```python
from build123d import *

# Parameters (mm, degrees)
EXTRUDE_1_DEPTH     = 10
SKETCH_2_W          = 10
SKETCH_2_H          = 510
EXTRUDE_2_DEPTH     = 500
EXTRUDE_3_DEPTH     = 10
EXTRUDE_4_DEPTH     = 190
SKETCH_5_W          = 640
SKETCH_5_H          = 10
EXTRUDE_5_DEPTH     = 200
CUT_EXTRUDE_1_DEPTH = 20
SKETCH_7_W          = 523.996532841
SKETCH_7_H          = 100
EXTRUDE_7_DEPTH     = 10
EXTRUDE_8_DEPTH     = 100
EXTRUDE_9_DEPTH     = 10
EXTRUDE_10_DEPTH    = 10
SKETCH_11_W         = 810
SKETCH_11_H         = 510
EXTRUDE_11_DEPTH    = 10
SKETCH_12_W         = 520
SKETCH_12_H         = 510
CUT_EXTRUDE_2_DEPTH = 120
SKETCH_13_W         = 520
SKETCH_13_H         = 510
CUT_EXTRUDE_3_DEPTH = 50
EXTRUDE_12_DEPTH    = 10
SKETCH_15_W         = 520
SKETCH_15_H         = 510
EXTRUDE_13_DEPTH    = 10
EXTRUDE_15_DEPTH    = 100
SKETCH_18_W         = 660
SKETCH_18_H         = 520
SKETCH_18_W_2       = 640
SKETCH_18_H_2       = 500
EXTRUDE_16_DEPTH    = 120
SKETCH_19_W         = 400
SKETCH_19_H         = 12
EXTRUDE_17_DEPTH    = 480
SKETCH_20_W         = 330
SKETCH_20_H         = 15
EXTRUDE_18_DEPTH    = 230


with BuildPart() as part:
    # 草图1 → 凸台-拉伸1 (new body)
    with BuildSketch(Plane(origin=(0, 0, 0), x_dir=(1, 0, 0), z_dir=(0, 1, 0))):
        Polygon((0, 300), (0, 510), (160, 510), (160, 320), (800, 320), (800, 0), (0, 0), align=None)
    extrude(amount=EXTRUDE_1_DEPTH)

    # 草图2 → 凸台-拉伸2 (add)
    with BuildSketch(Plane(origin=(0, 10, 0), x_dir=(1, 0, 0), z_dir=(0, 1, 0))):
        with Locations((5, 255)):
            Rectangle(SKETCH_2_W, SKETCH_2_H)
    extrude(amount=EXTRUDE_2_DEPTH)

    # 草图3 → 凸台-拉伸3 (add)
    with BuildSketch(Plane(origin=(0, 0, -510), x_dir=(-1, 0, 0), z_dir=(0, 0, -1))):
        Polygon((-10, 510), (-10, 10), (-160, 10), (-450.008667897, 510), align=None)
    extrude(amount=-EXTRUDE_3_DEPTH)

    # 草图4 → 凸台-拉伸4 (add)
    with BuildSketch(Plane(origin=(0, 0, -510), x_dir=(-1, 0, 0), z_dir=(0, 0, -1))):
        Polygon((-276.003467159, 210), (-160, 10), (-160, 0), (-169.762228515, 0), (-169.762228515, 10), (-285.765695674, 210), align=None)
    extrude(amount=-EXTRUDE_4_DEPTH)

    # 草图5 → 凸台-拉伸5 (add)
    with BuildSketch(Plane(origin=(0, 10, 0), x_dir=(1, 0, 0), z_dir=(0, 1, 0))):
        with Locations((480, 315)):
            Rectangle(SKETCH_5_W, SKETCH_5_H)
    extrude(amount=EXTRUDE_5_DEPTH)

    # 草图6 → 切除-拉伸1 (cut)
    with BuildSketch(Plane(origin=(0, 0, -320), x_dir=(-1, 0, 0), z_dir=(0, 0, -1))):
        Polygon((-160, 210), (-276.003467159, 210), (-160, 10), align=None)
    extrude(amount=-CUT_EXTRUDE_1_DEPTH, mode=Mode.SUBTRACT)

    # 草图7 → 凸台-拉伸7 (add)
    with BuildSketch(Plane(origin=(0, 210, 0), x_dir=(1, 0, 0), z_dir=(0, 1, 0))):
        with Locations((538.00173358, 360)):
            Rectangle(SKETCH_7_W, SKETCH_7_H)
    extrude(amount=-EXTRUDE_7_DEPTH)

    # 草图8 → 凸台-拉伸8 (add)
    with BuildSketch(Plane(origin=(0, 0, -510), x_dir=(-1, 0, 0), z_dir=(0, 0, -1))):
        Polygon((-276.003467159, 210), (-450.008667897, 510), (-459.770896412, 510), (-285.765695674, 210), align=None)
    extrude(amount=-EXTRUDE_8_DEPTH)

    # 草图9 → 凸台-拉伸9 (add)
    with BuildSketch(Plane.XY.offset(-410)):
        Polygon((276.003467159, 210), (450.008667897, 510), (800, 510), (800, 210), align=None)
    extrude(amount=EXTRUDE_9_DEPTH)

    # 草图10 → 凸台-拉伸10 (add)
    with BuildSketch(Plane(origin=(800, 0, 0), x_dir=(0, 0, -1), z_dir=(1, 0, 0))):
        Polygon((0, 0), (320, 0), (320, 200), (410, 200), (410, 510), (0, 510), align=None)
    extrude(amount=EXTRUDE_10_DEPTH)

    # 草图11 → 凸台-拉伸11 (add)
    with BuildSketch(Plane.XY):
        with Locations((405, 255)):
            Rectangle(SKETCH_11_W, SKETCH_11_H)
    extrude(amount=EXTRUDE_11_DEPTH)

    # 草图12 → 切除-拉伸2 (cut)
    with BuildSketch(Plane.ZY):
        with Locations((-250, 255)):
            Rectangle(SKETCH_12_W, SKETCH_12_H)
    extrude(amount=-CUT_EXTRUDE_2_DEPTH, mode=Mode.SUBTRACT)

    # 草图13 → 切除-拉伸3 (cut)
    with BuildSketch(Plane(origin=(810, 0, 0), x_dir=(0, 0, -1), z_dir=(1, 0, 0))):
        with Locations((250, 255)):
            Rectangle(SKETCH_13_W, SKETCH_13_H)
    extrude(amount=-CUT_EXTRUDE_3_DEPTH, mode=Mode.SUBTRACT)

    # 草图14 → 凸台-拉伸12 (add)
    with BuildSketch(Plane(origin=(760, 0, 0), x_dir=(0, 0, -1), z_dir=(1, 0, 0))):
        Polygon((-10, 510), (320, 510), (410, 510), (410, 200), (320, 200), (320, 0), (-10, 0), align=None)
    extrude(amount=EXTRUDE_12_DEPTH)

    # 草图15 → 凸台-拉伸13 (add)
    with BuildSketch(Plane.ZY.offset(-120)):
        with Locations((-250, 255)):
            Rectangle(SKETCH_15_W, SKETCH_15_H)
    extrude(amount=EXTRUDE_13_DEPTH)

    # 草图17 → 凸台-拉伸15 (add)
    with BuildSketch(Plane(origin=(0, 0, -410), x_dir=(-1, 0, 0), z_dir=(0, 0, -1))):
        Polygon((-770, 510), (-459.770896412, 510), (-453.970723054, 500), (-770, 500), align=None)
    extrude(amount=EXTRUDE_15_DEPTH)

    # 草图18 → 凸台-拉伸16 (add)
    with BuildSketch(Plane(origin=(0, 510, 0), x_dir=(1, 0, 0), z_dir=(0, 1, 0))):
        with Locations((440, 250)):
            Rectangle(SKETCH_18_W, SKETCH_18_H)
        with Locations((440, 250)):
            Rectangle(SKETCH_18_W_2, SKETCH_18_H_2, mode=Mode.SUBTRACT)
    extrude(amount=EXTRUDE_16_DEPTH)

    # 草图19 → 凸台-拉伸17 (add)
    with BuildSketch(Plane.ZY.offset(-110)):
        with Locations((-250, 506)):
            Rectangle(SKETCH_19_W, SKETCH_19_H)
    extrude(amount=EXTRUDE_17_DEPTH)

    # 草图20 → 凸台-拉伸18 (add)
    with BuildSketch(Plane(origin=(770, 0, 0), x_dir=(0, 0, -1), z_dir=(1, 0, 0))):
        with Locations((155, 207.5)):
            Rectangle(SKETCH_20_W, SKETCH_20_H)
    extrude(amount=EXTRUDE_18_DEPTH)


solid = part.part
```
Verification items for the finished model (mm, model axes). A direction names the side the tool comes from. Give positions to 0.01 mm unless a question says otherwise; leave off trailing zeros. Write each loop counter-clockwise with the first axis right and the second up, starting at its lowest first coordinate (ties: lowest second). Pieces come first, ordered by that corner, then holes. Notation, with made-up numbers: M -32.75,49.5 L 20.25,49.5 A13 cw 20.25,58.5 Z; hole C 45.5,-30 d8. An arc over 180 degrees is marked long. One line per question, with ' | ' between items.
1) Set-up check for faces 1 (the flat face through (607, 510, -449)), 2 (the flat face through (-127, 500, -253)), 3 (the flat face through (-127, 512, -253)), 4 (the flat face through (576, 352, -410)), 5 (the flat face through (883, 215, -153)): record each of +Z, -Z, +X, -X, +Y, -Y from which the full face is reachable in a straight line by a thin tool's end or side.
Result:
face 1: +Y | face 2: +Z, -Z, -X, -Y | face 3: +Z, -Z, -X, +Y | face 4: -Z, +X, -Y | face 5: +Z, -Z, +X, +Y
2) Mould release check, pull along X, two halves, no side actions. Record for faces 6 (the flat face through (575, 362, -400)), 7 (the flat face through (466, 101, -320)): released by +X, released by -X, zero draft, split by the parting line, or undercut.
Result:
face 6: undercut | face 7: zero draft
3) Section check D-D on z = -138.5. Enter the section's corners in (x, y), plus the area to 3 significant figures.
Result:
outline: M -370,500 L 110,500 L 110,0 L 770,0 L 770,200 L 1000,200 L 1000,215 L 770,215 L 770,630 L 760,630 L 760,10 L 120,10 L 120,630 L 110,630 L 110,512 L -370,512 Z | area: 28,200 mm2
4) Gauge pin test, flat ends, axial feed: pin 1 Ø2 at (x, z) = (-185.5, -178) entering from -Y; pin 2 Ø5 at (y, z) = (475, -168.5) entering from -X; pin 3 Ø9.5 at (x, y) = (-167, 504.5) entering from +Z; pin 4 Ø2 at (x, z) = (226.5, -175) entering from -Y. Record the tip position at first contact, or that the pin passes through.
Result:
pin 1: stops at y = 500 | pin 2: stops at x = 110 | pin 3: stops at z = -50 | pin 4: stops at y = 0
5) Section check A-A on z = -364.5. Enter the section's corners in (x, y).
Result:
outline: M -370,500 L 110,500 L 110,0 L 169.76,0 L 169.76,10 L 279.97,200 L 770,200 L 770,630 L 760,630 L 760,210 L 276,210 L 160,10 L 120,10 L 120,630 L 110,630 L 110,512 L -370,512 Z
6) Thickness scan on line 1 along X through (y, z) = (305.5, -143); line 2 along Z through (x, y) = (415.5, 339); line 3 along Z through (x, y) = (129, 409). Record the ranges inside material, lowest first. Write a range as [from, to].
Result:
line 1: x = [110, 120], [760, 770] | line 2: z = [-410, -400], [0, 10] | line 3: z = [-510, -500], [0, 10]
7) Section check B-B on y = 434. Enter the section's corners in (x, z), plus the area to 3 significant figures.
Result:
outline: M 110,-510 L 415.69,-510 L 415.69,-410 L 770,-410 L 770,10 L 110,10 Z; hole M 120,-500 L 405.93,-500 L 405.93,-400 L 760,-400 L 760,0 L 120,0 Z | area: 23,200 mm2
8) Section check C-C on x = 379.5. Enter the section's corners in (y, z).
Result:
outline: M 0,-320 L 200,-320 L 200,-410 L 371.61,-410 L 371.61,-510 L 630,-510 L 630,-500 L 388.44,-500 L 388.44,-400 L 210,-400 L 210,-310 L 10,-310 L 10,0 L 630,0 L 630,10 L 0,10 Z
